```python
from build123d import *

# Parameters (mm, degrees)
F0_W     = 203.2
F0_H     = 203.2
F1_DEPTH = 19.05
F3_D     = 9.525
F4_R     = 12.6365
F5_DEPTH = 254


# Not quite as in the source:
# - a length typed as a fraction of an inch, garbled in the dataset ("3 / 203.2 mm" for 3/8 in), is restored


with BuildPart() as f1:
    # F0 (on Top) → F1 (new body)
    with BuildSketch(Plane.XY):
        Rectangle(F0_W, F0_H)
    extrude(amount=F1_DEPTH)

    # F3 (through all)
    with Locations(Plane.XY.offset(19.05)):
        with Locations((-77.7875, 76.2), (77.7875, 76.2), (-77.7875, -76.2), (77.7875, -76.2)):
            Hole(F3_D / 2)

    # F4 (on face) → F5 (join)
    with BuildSketch(Plane.XY.offset(19.05)):
        Circle(F4_R)
    extrude(amount=F5_DEPTH)


solid = f1.part
```
CAD build for the part. Positions are in the model's coordinates, mm. Give positions to 0.01 mm unless a question says otherwise; leave off trailing zeros. Loops run counter-clockwise (first coordinate to the right, second up) from the corner with the lowest first, then second, coordinate; pieces in that order, holes last. Notation, with made-up numbers: M 74,-13.75 L 118,-13.75 A4 cw 118,-7.75 Z; hole C 19.5,37.5 d10. An arc over 180 degrees is marked long. Use one line per item in the form item = value.
Item 1: Two-plate mould, pull along Y, no slides. Class faces 1 (the face through (5.83, -11.21, 144.27)), 2 (the face through (-77.168, -71.478, 9.392)), 3 (the face through (101.6, -1, 9)): pulls with the +Y half, pulls with the -Y half, needs draft (parallel to the pull), parting line crosses it, or undercut.
Determined:
face_1 = parting line crosses it
face_2 = undercut
face_3 = needs draft
Item 2: Slice it at A-A (y = 76.2). List the corners of the cut face in (x, z) (3 decimals).
Determined:
outline = M -101.6,0 L -82.55,0 L -82.55,19.05 L -101.6,19.05 Z; M -73.025,0 L 73.025,0 L 73.025,19.05 L -73.025,19.05 Z; M 82.55,0 L 101.6,0 L 101.6,19.05 L 82.55,19.05 Z
Item 3: Flat gauge pins, fed straight in: pin 1 (7.5 mm diameter, centred on x = -77.79, y = -76.2, fed in from -Z); pin 2 (12 mm diameter, centred on x = -16, y = -76, fed in from +Z). Where does each tip first touch, or does it go through?
Determined:
pin_1 = through
pin_2 = 19.05
Item 4: Slice it at B-B (x = 0). List the corners of the cut face in (y, z).
Determined:
outline = M -101.6,0 L 101.6,0 L 101.6,19.05 L 12.64,19.05 L 12.64,273.05 L -12.64,273.05 L -12.64,19.05 L -101.6,19.05 Z
Item 5: Slice it at D-D (z = 171). List the corners of the cut face in (x, y).
Determined:
outline = C 0,0 d25.27
Item 6: Drill centre lines: probe 1 along Z at (x, y) = (-10.5, -83); probe 2 along Y at (x, z) = (6.5, 234); probe 3 along X at (y, z) = (-3, 116.5). Where is each one in solid material? Low to high. Write a range as from..to.
Determined:
probe_1 = 0..19.05
probe_2 = -10.84..10.84
probe_3 = -12.28..12.28
